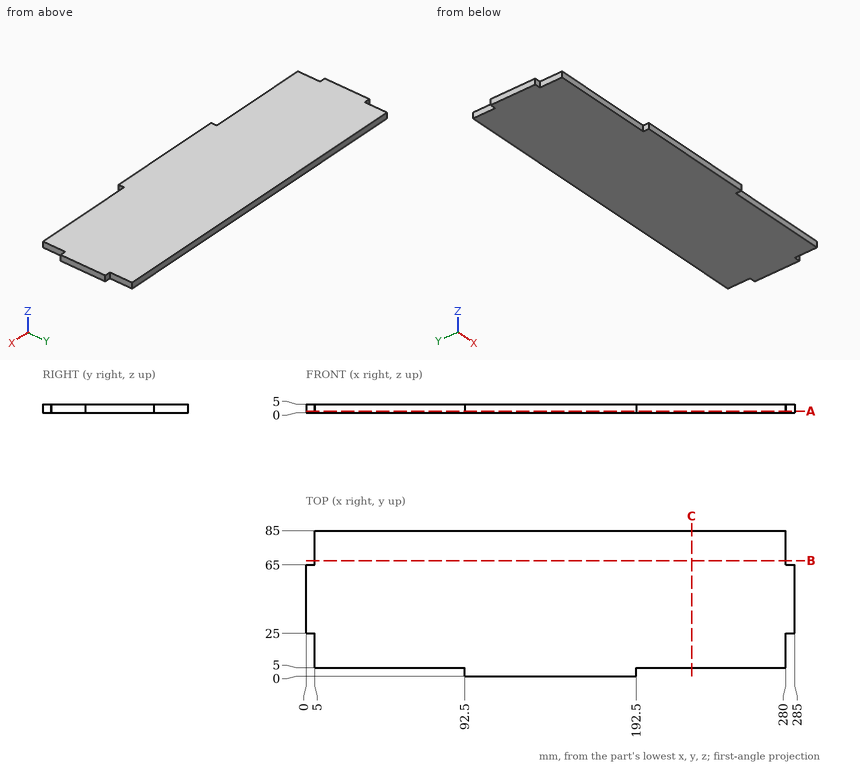
Check sheet for the drawn part. Datum: minimum x, y, z corner. Units: mm. Coordinates: 2 decimals unless noted, no trailing zeros. Order: outer loops, then holes, each group sorted by start corner. A loop starts at its lowest first (then second) coordinate and runs counter-clockwise, first axis right, second up. Notation, with made-up numbers: M -40,65.5 L -25,65.5 A13 ccw -25,72.5 Z; hole C 36,24 d8. An arc over 180 degrees is marked long. One line per question, with ' | ' between items. Start each with the question number.
Item 1: Cross-section at C-C on x = 225. Enter the section's corners in (y, z).
Item 2: Gauge pin test, flat ends, axial feed: pin 1 (2.5 mm diameter, centred on y = 11, z = 3, fed in from -X); pin 2 (2 mm diameter, centred on y = 11.5, z = 3.5, fed in from +X); pin 3 (2.5 mm diameter, centred on x = 282.5, z = 1.5, fed in from -Y). Record the tip position at first contact, or that the pin passes through.
Item 3: Cross-section at A-A on z = 0.8. Enter the section's corners in (x, y), then the cut area to 3 significant figures.
Item 4: Cross-section at B-B on y = 67.5. Enter the section's corners in (x, z), then the cut area to 4 significant figures.
Item 5: Material ranges on L1, parallel to Y at x = 24, z = 2.5; L2, parallel to X at y = 23.5, z = 1.35, recorded low to high. Write a range as [from, to].
Findings:
1) outline: M 5,0 L 85,0 L 85,5 L 5,5 Z
2) pin 1: stops at x = 5 | pin 2: stops at x = 280 | pin 3: stops at y = 25
3) outline: M 0,25 L 5,25 L 5,5 L 92.5,5 L 92.5,0 L 192.5,0 L 192.5,5 L 280,5 L 280,25 L 285,25 L 285,65 L 280,65 L 280,85 L 5,85 L 5,65 L 0,65 Z | area: 22,900 mm²
4) outline: M 5,0 L 280,0 L 280,5 L 5,5 Z | area: 1,375 mm²
5) L1: y = [5, 85] | L2: x = [5, 280]
